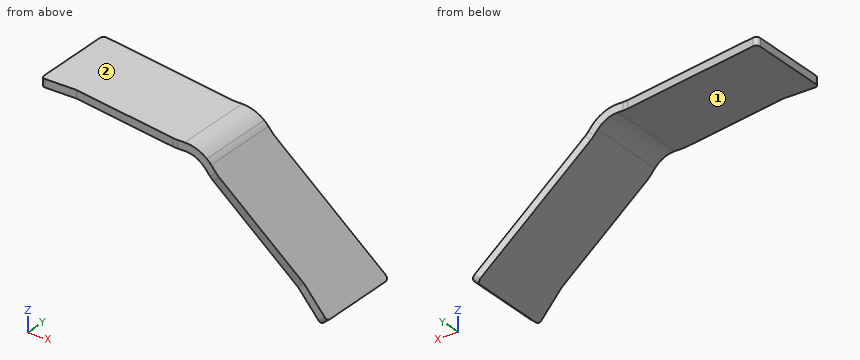
from build123d import *

# Parameters (mm, degrees)
BASE_EXTRUDE_DEPTH     = 6
PROCESS_BENDS1_START   = -47.212369611
PROCESS_BENDS1_DEPTH   = 79.424739222
PROCESS_BENDS1_START_2 = -29.212369611
PROCESS_BENDS1_2_DEPTH = 42
PROCESS_BENDS1_3_DEPTH = 79.379162481
PROCESS_BENDS1_START_3 = -7.599506721
PROCESS_BENDS1_4_DEPTH = 13.144247807
PROCESS_BENDS1_START_4 = -0.455258914
PROCESS_BENDS1_5_DEPTH = 6


with BuildPart() as part:
    # Sketch1 → Base-Extrude (new body)
    with BuildSketch(Plane.XY):
        with BuildLine():
            Line((-125.479055467, 32.16679287), (-17.29755389, 13.091475329))
            ThreePointArc((-17.29755389, 13.091475329), (-15.567705192, 12.863736427), (-13.824590337, 12.787630389))
            Line((-13.824590337, 12.787630389), (13.824590337, 12.787630389))
            ThreePointArc((13.824590337, 12.787630389), (15.567705192, 12.863736427), (17.29755389, 13.091475329))
            Line((17.29755389, 13.091475329), (125.479055467, 32.16679287))
            ThreePointArc((125.479055467, 32.16679287), (127.928362829, 31.51050294), (129, 29.212369611))
            Line((129, 29.212369611), (129, -29.212369611))
            ThreePointArc((129, -29.212369611), (128.121320344, -31.333689955), (126, -32.212369611))
            Line((126, -32.212369611), (102.366781185, -32.212369611))
            Line((102.366781185, -32.212369611), (19.020744173, -46.908524671))
            ThreePointArc((19.020744173, -46.908524671), (17.290895475, -47.136263573), (15.54778062, -47.212369611))
            Line((15.54778062, -47.212369611), (-15.54778062, -47.212369611))
            ThreePointArc((-15.54778062, -47.212369611), (-17.290895475, -47.136263573), (-19.020744173, -46.908524671))
            Line((-19.020744173, -46.908524671), (-102.366781185, -32.212369611))
            Line((-102.366781185, -32.212369611), (-126, -32.212369611))
            ThreePointArc((-126, -32.212369611), (-128.121320344, -31.333689955), (-129, -29.212369611))
            Line((-129, -29.212369611), (-129, 29.212369611))
            ThreePointArc((-129, 29.212369611), (-127.928362829, 31.51050294), (-125.479055467, 32.16679287))
        make_face()
    extrude(amount=BASE_EXTRUDE_DEPTH)

    # Process-Bends1: read off the stored shape, not the designer's step
    # Process-Bends1 outline → Process-Bends1 (cut)
    with BuildSketch(Plane(origin=(0, 0, 0), x_dir=(1, 0, 0), z_dir=(0, 1, 0)).offset(PROCESS_BENDS1_START)):
        with BuildLine():
            Line((129, 0), (6.692796258, 0))
            ThreePointArc((6.692796258, 0), (-1.088690602, -4.454038521), (-9.920451468, -6))
            Line((-9.920451468, -6), (129, -6))
            Line((129, -6), (129, 0))
        make_face()
    extrude(amount=PROCESS_BENDS1_DEPTH, mode=Mode.SUBTRACT)

    # Process-Bends1 2 outline → Process-Bends1 2 (add)
    with BuildSketch(Plane(origin=(0, 0, 0), x_dir=(1, 0, 0), z_dir=(0, 1, 0)).offset(PROCESS_BENDS1_START_2)):
        with BuildLine():
            ThreePointArc((6.692796258, 0), (8.418565431, 1.569577889), (9.996704053, 3.287522148))
            Line((9.996704053, 3.287522148), (86.539562416, 94.50774859))
            Line((86.539562416, 94.50774859), (81.943295757, 98.364474248))
            Line((81.943295757, 98.364474248), (5.400437394, 7.144247806))
            ThreePointArc((5.400437394, 7.144247806), (-1.468086233, 1.873844259), (-9.920451468, 0))
            Line((-9.920451468, 0), (6.692796258, 0))
        make_face()
    extrude(amount=PROCESS_BENDS1_2_DEPTH)

    # Process-Bends1 3 outline → Process-Bends1 3 (add)
    with BuildSketch(Plane(origin=(0, 0, 0), x_dir=(1, 0, 0), z_dir=(0, 1, 0)).offset(PROCESS_BENDS1_START)):
        with BuildLine():
            ThreePointArc((6.692796258, 0), (8.418565431, 1.569577889), (9.996704053, 3.287522148))
            Line((9.996704053, 3.287522148), (86.539562416, 94.50774859))
            Line((86.539562416, 94.50774859), (81.943295757, 98.364474248))
            Line((81.943295757, 98.364474248), (5.400437394, 7.144247806))
            ThreePointArc((5.400437394, 7.144247806), (-1.468086233, 1.873844259), (-9.920451468, 0))
            Line((-9.920451468, 0), (6.692796258, 0))
        make_face()
    extrude(amount=PROCESS_BENDS1_3_DEPTH)

    # Process-Bends1 4 outline → Process-Bends1 4 (cut)
    with BuildSketch(Plane(origin=(0, 0, 0), x_dir=(0.6427876096865379, 0, -0.7660444431189791), z_dir=(0.7660444431189791, 0, 0.6427876096865381)).offset(PROCESS_BENDS1_START_3)):
        with BuildLine():
            Line((-8, 12.787630389), (12.848284445, 12.787630389))
            ThreePointArc((12.848284445, 12.787630389), (14.5913993, 12.863736427), (16.321247998, 13.091475329))
            Line((16.321247998, 13.091475329), (124.502749575, 32.16679287))
            Line((124.502749575, 32.16679287), (-8, 32.16679287))
            Line((-8, 32.16679287), (-8, 12.787630389))
        make_face()
        with BuildLine():
            Line((128.023694108, 32.16679287), (125.54463864, 32.16679287))
            ThreePointArc((125.54463864, 32.16679287), (127.321827437, 31.14073244), (128.023694108, 29.212369611))
            Line((128.023694108, 29.212369611), (128.023694108, 32.16679287))
        make_face()
        with BuildLine():
            ThreePointArc((18.044438281, -46.908524671), (16.314589583, -47.136263573), (14.571474728, -47.212369611))
            Line((14.571474728, -47.212369611), (128.023694108, -47.212369611))
            Line((128.023694108, -47.212369611), (128.023694108, -29.212369611))
            ThreePointArc((128.023694108, -29.212369611), (127.145014451, -31.333689954), (125.023694108, -32.212369611))
            Line((125.023694108, -32.212369611), (101.390475292, -32.212369611))
            Line((101.390475292, -32.212369611), (18.044438281, -46.908524671))
        make_face()
    extrude(amount=PROCESS_BENDS1_4_DEPTH, mode=Mode.SUBTRACT)

    # Process-Bends1 5 outline → Process-Bends1 5 (add)
    with BuildSketch(Plane(origin=(0, 0, 0), x_dir=(0.6427876096865379, 0, -0.7660444431189791), z_dir=(0.7660444431189791, 0, 0.6427876096865381)).offset(PROCESS_BENDS1_START_4)):
        with BuildLine():
            ThreePointArc((125.54463864, 32.16679287), (125.023694107, 32.212369611), (124.502749575, 32.16679287))
            Line((124.502749575, 32.16679287), (125.54463864, 32.16679287))
        make_face()
    extrude(amount=PROCESS_BENDS1_5_DEPTH)


solid = part.part
The listing builds one solid part. Answer for the finished solid, in the listing's coordinates (mm). Face numbers are marked on the shaded views. A direction names the side the tool comes from. Round coordinates to 2 decimals unless told otherwise and drop trailing zeros. Order: outer loops, then holes, each group sorted by start corner. A loop starts at its lowest first (then second) coordinate and runs counter-clockwise, first axis right, second up. Notation, with made-up numbers: M 40,53 L 61,53 A31 cw 61,89 Z; hole C -19.75,-22.75 d5. An arc over 180 degrees is marked long. Answer in a Markdown table with one row per item. Add a question column.
1) The part is cut by section A-A on y = 24. Determine the outline of the cut face in (x, z), plus the area to 3 significant figures.
2) Which of the six approach directions +Z, -Z, +X, -X, +Y, -Y give full straight-line access (tool end or side, diameter ignored) to the marked faces 1 and 2?
3) The part is cut by section C-C on z = -39.5. Determine the outline of the cut face in (x, y).
4) The part is cut by section D-D on x = -4. Determine the outline of the cut face in (y, z), plus the area to 3 significant figures.
5) Consider line 1 along Z through (x, y) = (-15, 9.5); line 2 along Z through (x, y) = (27, -3); line 3 along X through (y, z) = (21.5, -62). Determine where each line is inside the solid, lowest interval first. Write a range as from..to.
6) The part is cut by section B-B on y = -23. Determine the outline of the cut face in (x, z), plus the area to 3 significant figures.
7) Flat-ended cylindrical pins translate along their axes: pin 1 Ø1 at (y, z) = (-18.5, -26.5) entering from +X; pin 2 Ø3 at (y, z) = (-5.5, -48.5) entering from +X; pin 3 Ø3 at (x, z) = (-114.5, 3) entering from -Y. Find the tip coordinate at first contact, or state that the pin passes through.
Findings below:
| question | item | result |
|---|---|---|
| 1 | outline | M -129,0 L -79.16,0 L -79.16,6 L -129,6 Z; M 49.91,-60.19 L 81.94,-98.36 L 86.54,-94.51 L 54.5,-56.33 Z |
| 1 | area | 598 mm² |
| 2 | face 1 | -Z, -X, +Y, -Y |
| 2 | face 2 | +Z, +X, -X, +Y, -Y |
| 3 | outline | M 32.55,-41.07 L 40.38,-40.18 L 40.38,20.13 L 32.55,19.24 Z |
| 4 | outline | M -47.21,-0.9 L 12.79,-0.9 L 12.79,5.32 L -47.21,5.32 Z |
| 4 | area | 373 mm² |
| 5 | line 1 | z = 0..6 |
| 5 | line 2 | z = -32.89..-23.55 |
| 5 | line 3 | x = 51.43..59.26 |
| 6 | outline | M -129,0 L -9.92,0 A20 cw 5.4,-7.14 L 81.94,-98.36 L 86.54,-94.51 L 10,-3.29 A26 ccw -9.92,6 L -129,6 Z |
| 6 | area | 1,550 mm² |
| 7 | pin 1 | stops at x = 29.89 |
| 7 | pin 2 | stops at x = 49.19 |
| 7 | pin 3 | stops at y = -32.21 |
